Geometry check sheet. Reference: the model listing, model coordinates, mm. A direction names the side the tool comes from. Coordinates: 2 decimals unless noted, no trailing zeros. Write each loop counter-clockwise with the first axis right and the second up, starting at its lowest first coordinate (ties: lowest second). Pieces come first, ordered by that corner, then holes. Notation, with made-up numbers: (-1.75, 25) -> (11.25, 25) arc R32 cw to (11.25, 59) -> close; hole circle Ø3 at (67.25, 71). An arc over 180 degrees is marked (long way). Answer in a Markdown table with one row per item. Add a question column.
Q1. Section check C-C, the plane x = 8.25. Record the boundary of the cut face in (y, z).
Q2. Release check for a two-part mould opening along X. For faces 3 (the face through (-0.5, 23.4, 25)), 4 (the face through (0.5, 35, 13)), 5 (the face through (-1, 34, 12)) record: pulls with the +X half, pulls with the -X half, needs draft (parallel to the pull), parting line crosses it, or undercut.
Q3. Section check A-A, the plane y = 45. Record the boundary of the cut face in (x, z), and give its area (4 significant figures).
Q4. Section check B-B, the plane z = 11. Record the boundary of the cut face in (x, y).
Q5. Thickness scan on line 1 (X direction, y = 10.5, z = 1.25); line 2 (Y direction, x = 18.5, z = 13.5). Record the ranges inside material, lowest first.
Q6. Tool access check on faces 1 (the face through (14, -1, 12)), 2 (the face through (27.5, 34, 13)). Record the directions out of +Z, -Z, +X, -X, +Y, -Y that give a thin tool (end or side, any length) a straight path to the whole face; none if there is none.
Q7. Gauge pin test, flat ends, axial feed: P1, Ø13.5, axis at x = 13.5, y = 42, coming from the +Z side; P2, Ø7.5, axis at x = 13, z = 9, coming from the +Y side. Record the tip position at first contact, or that the pin passes through.
Autodesk Fusion 360 part; units mm, degrees
sketch "Sketch1" plane through (0, 0, 0) normal (0, 0, 1) x (1, 0, 0)
  line L0 (0, 0) -> (28, 0)
  line L1 (28, 0) -> (28, 68)
  line L2 (28, 68) -> (0, 68)
  line L3 (0, 68) -> (0, 0)
  dimension "d1" = 28
  dimension "d2" = 68
extrude "Extrude1" add sketch "Sketch1" along normal blind 25
shell "Shell1" thickness 0.5 removed faces 2 at (18.6667, 68, 8.3333) at (9.3333, 45.3333, 25)
extrude "Extrude2" add 1 faces at (9.3333, 45.3333, 0) along direction (0, 0, -1) blind 1
extrude "Extrude3" add 1 faces at (28, 45.3333, 16.3333) along direction (1, 0, 0) blind 1
extrude "Extrude4" add 1 faces at (0, 45.3333, 7.6667) along direction (-1, 0, 0) blind 1
extrude "Extrude5" add 1 faces at (9, 0, 16.3333) along direction (0, -1, 0) blind 1
Calculated:
| question | item | result |
|---|---|---|
| 1 | outline | (-1, -1) -> (68, -1) -> (68, 0.5) -> (0.5, 0.5) -> (0.5, 25) -> (-1, 25) -> close |
| 2 | face 3 | needs draft |
| 2 | face 4 | undercut |
| 2 | face 5 | pulls with the -X half |
| 3 | outline | (-1, -1) -> (29, -1) -> (29, 25) -> (27.5, 25) -> (27.5, 0.5) -> (0.5, 0.5) -> (0.5, 25) -> (-1, 25) -> close |
| 3 | area | 118.5 mm² |
| 4 | outline | (-1, -1) -> (29, -1) -> (29, 68) -> (27.5, 68) -> (27.5, 0.5) -> (0.5, 0.5) -> (0.5, 68) -> (-1, 68) -> close |
| 5 | line 1 | x = -1 to 0.5, 27.5 to 29 |
| 5 | line 2 | y = -1 to 0.5 |
| 6 | face 1 | +Z, -Z, +X, -X, -Y |
| 6 | face 2 | +Z, +Y |
| 7 | P1 | stops at z = 0.5 |
| 7 | P2 | stops at y = 0.5 |
